from build123d import *

# Parameters (mm, degrees)
BOSS_EXTRUDE1_DEPTH = 10
SKETCH4_R           = 1.5
SKETCH4_R_2         = 0.8
CUT_EXTRUDE1_DEPTH  = 42
SKETCH6_R           = 0.8
CUT_EXTRUDE2_DEPTH  = 26
CUT_EXTRUDE3_DEPTH  = 2
SKETCH9_R           = 2.5
CUT_EXTRUDE4_DEPTH  = 10


with BuildPart() as part:
    # Sketch2 → Boss-Extrude1 (new body)
    with BuildSketch(Plane.XY):
        Polygon((-16.5, -11), (-19.5, -11), (-19.5, 14), (21.5, 14), (21.5, -11), (16.5, -11), (16.5, 11), (-16.5, 11), align=None)
    extrude(amount=BOSS_EXTRUDE1_DEPTH)

    # Sketch4 → Cut-Extrude1 (cut, through all)
    with BuildSketch(Plane.ZY.offset(19.5)):
        with Locations((5, -6)):
            Circle(SKETCH4_R)
        with Locations((5, -1)):
            Circle(SKETCH4_R_2)
    extrude(amount=-CUT_EXTRUDE1_DEPTH, mode=Mode.SUBTRACT)

    # Sketch6 → Cut-Extrude2 (cut, through all)
    with BuildSketch(Plane(origin=(0, 14, 0), x_dir=(1, 0, 0), z_dir=(0, 1, 0))):
        with Locations((-9, -5)):
            Circle(SKETCH6_R)
        with Locations((9, -5)):
            Circle(SKETCH6_R)
    extrude(amount=-CUT_EXTRUDE2_DEPTH, mode=Mode.SUBTRACT)

    # Sketch8 → Cut-Extrude3 (cut)
    with BuildSketch(Plane.ZY.offset(-16.5)):
        Polygon((1, -1), (1, -11), (9, -11), (9, -1), (7, 12), (3, 12), align=None)
    extrude(amount=-CUT_EXTRUDE3_DEPTH, mode=Mode.SUBTRACT)

    # Sketch9 → Cut-Extrude4 (cut)
    with BuildSketch(Plane.ZY.offset(19.5)):
        with Locations((5, -6)):
            Circle(SKETCH9_R)
    extrude(amount=-CUT_EXTRUDE4_DEPTH, mode=Mode.SUBTRACT)


solid = part.part
Here's how the part is built. I have some questions about the finished solid (model axes, mm). A direction names the side the tool comes from. Coordinates: 2 decimals unless noted, no trailing zeros. Loops run counter-clockwise (first coordinate to the right, second up) from the corner with the lowest first, then second, coordinate; pieces in that order, holes last.
1. For faces 1 (the cylindrical face through (-18.021, -5.249, 7.385)), 2 (the flat face through (16.5, 2, 1)), 3 (the flat face through (17.486, 5.591, 2.014)), 4 (the flat face through (4, 12, 0)), which set-ups out of +Z, -Z, +X, -X, +Y, -Y let a thin tool reach every point of the face, with its end or its side?
2. If we mould it in two halves opening along X, with no side actions, what happens to faces 5 (the cylindrical face through (19.979, -6.575, 6.386)), 6 (the cylindrical face through (8.83, 12.52, 5.78)), 7 (the flat face through (0, 11, 5)), 8 (the flat face through (-19.5, 1, 5))? For each: pulls with the +X half, pulls with the -X half, needs draft (parallel to the pull), parting line crosses it, or undercut.
3. Imagine slicing it at B-B, the plane z = 5. Count the separate pieces of the cut face and the enclosed holes in it, and give its area (3 significant figures).
4. I need wall thicknesses on L1, parallel to X at y = 13.4, z = 5; L2, parallel to X at y = 3, z = 0.5; L3, parallel to Z at x = -9, y = 13.35. Which ranges of each line are inside material? Lowest first, please.
5. Imagine slicing it at D-D, the plane y = 3.75. Please give me the cut outline in (x, z), and give its area (3 significant figures).
6. For P1, Ø1.8, axis at x = 9, z = 5, coming from the -Y side, with a flat end and sliding along its axis, tell me the tip position at first contact or that it passes through.
7. Imagine slicing it at A-A, the plane x = 9. Please give me the cut outline in (y, z), and give its area (3 significant figures).
8. Imagine slicing it at C-C, the plane y = -6.5. Please give me the cut outline in (x, z), and give its area (3 significant figures).
Taken from the geometry:
1. face 1: -X
1. face 2: +Z, -Z, -Y
1. face 3: -Y
1. face 4: -Z, +X, -X, +Y, -Y
2. face 5: needs draft
2. face 6: undercut
2. face 7: undercut
2. face 8: pulls with the -X half
3. separate pieces: 7
3. enclosed holes: 0
3. area: 210 mm2
4. L1: x = -19.5 to -9.8, -8.2 to 8.2, 9.8 to 21.5
4. L2: x = -19.5 to -16.5, 16.5 to 21.5
4. L3: z = 0 to 4.2, 5.8 to 10
5. outline: (-19.5, 0) - (-16.5, 0) - (-16.5, 10) - (-19.5, 10) - close; (16.5, 0) - (21.5, 0) - (21.5, 10) - (16.5, 10) - (16.5, 8.27) - (18.5, 8.27) - (18.5, 1.73) - (16.5, 1.73) - close
5. area: 66.9 mm2
6. P1: stops at y = 11
7. outline: (11, 0) - (14, 0) - (14, 4.2) - (11, 4.2) - close; (11, 5.8) - (14, 5.8) - (14, 10) - (11, 10) - close
7. area: 25.2 mm2
8. outline: (-19.5, 0) - (-16.5, 0) - (-16.5, 2.55) - (-19.5, 2.55) - close; (-19.5, 7.45) - (-16.5, 7.45) - (-16.5, 10) - (-19.5, 10) - close; (16.5, 0) - (21.5, 0) - (21.5, 3.59) - (18.5, 3.59) - (18.5, 1) - (16.5, 1) - close; (16.5, 9) - (18.5, 9) - (18.5, 6.41) - (21.5, 6.41) - (21.5, 10) - (16.5, 10) - close
8. area: 40.8 mm2
